Geometry check sheet. Reference: drawing and pictorial views, mm from the part's lowest x, y, z. A direction names the side the tool comes from. Coordinates: 2 decimals unless noted, no trailing zeros. Write each loop counter-clockwise with the first axis right and the second up, starting at its lowest first coordinate (ties: lowest second). Pieces come first, ordered by that corner, then holes. Notation, with made-up numbers: (45.5, 40) - (87.5, 40) arc R20 ccw to (87.5, 47) - close; hole circle Ø1 at (30.25, 74.25). An arc over 180 degrees is marked (long way). Answer as a JSON object with one key per item and string values. Group by question number.
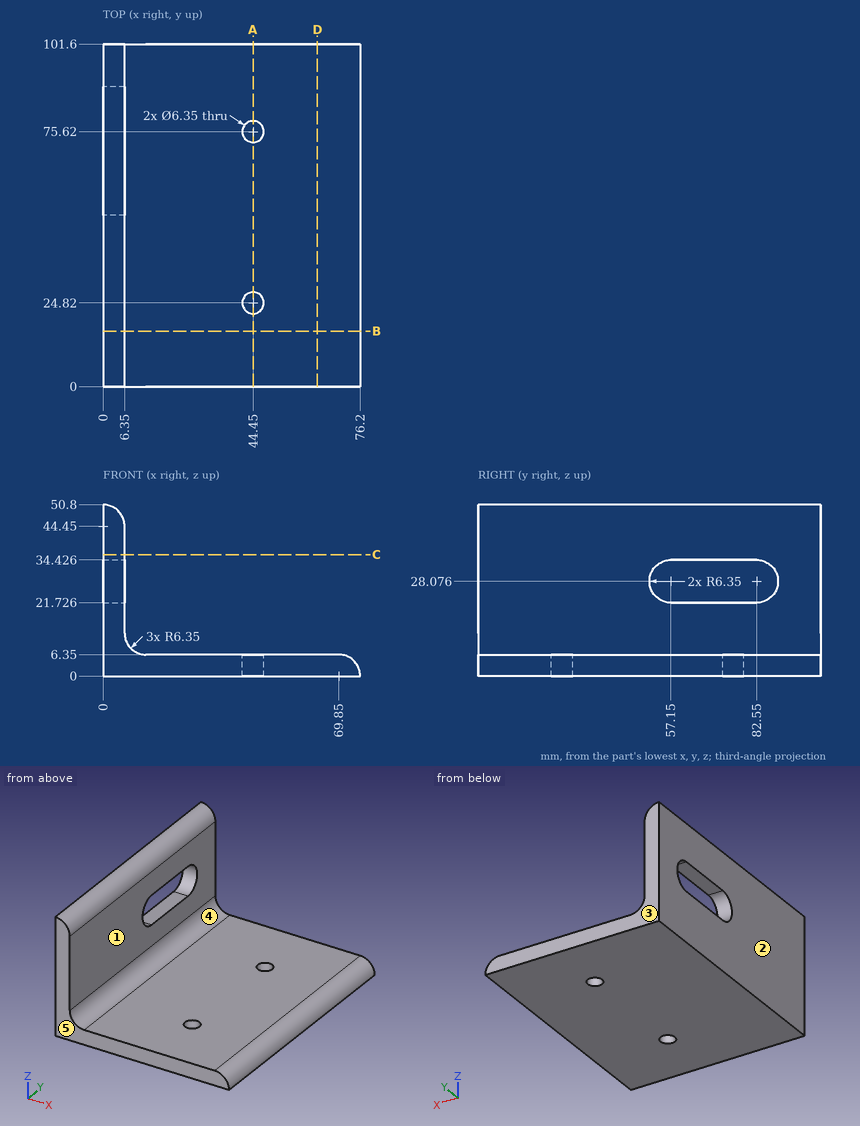
(1) Material ranges on L1, parallel to Y at x = 44.45, z = 4 (1 decimal); L2, parallel to X at y = 10.5, z = 17.5; L3, parallel to Z at x = 5.5, y = 43 (1 decimal), recorded low to high. Write a range as [from, to].
(2) Section check B-B (y = 16.5). Record the cut outline in (x, z).
(3) Section check C-C (z = 36). Record the cut outline in (x, y), and give its area (3 significant figures).
(4) Draft check along Y on the marked faces 3, 4 and 5. Enter one of: +Y half, -Y half, draft (parallel to the pull), parting line (faces both ways), or undercut.
(5) Section check D-D (x = 63.5). Record the cut outline in (y, z).
(6) Section check A-A (x = 44.45). Count the separate pieces of the cut face and the enclosed holes in it.
(7) Set-up check for the marked faces 1 and 2: record each of +Z, -Z, +X, -X, +Y, -Y from which the full face is reachable in a straight line by a thin tool's end or side.
(8) Gauge pin test, flat ends, axial feed: pin 1 (2 mm diameter, centred on x = 22.5, y = 34, fed in from +Z); pin 2 (4 mm diameter, centred on y = 89.5, z = 11, fed in from +X); pin 3 (5 mm diameter, centred on x = 3, y = 75.5, fed in from +Z). Record the tip position at first contact, or that the pin passes through.
Conclusion:
{
 "1": {"L1": "y = [0, 21.6], [28, 72.4], [78.8, 101.6]", "L2": "x = [0, 6.35]", "L3": "z = [0, 47.6]"},
 "2": {"outline": "(0, 0) - (76.2, 0) arc R6.35 ccw to (69.85, 6.35) - (12.7, 6.35) arc R6.35 cw to (6.35, 12.7) - (6.35, 44.45) arc R6.35 ccw to (0, 50.8) - close"},
 "3": {"outline": "(0, 0) - (6.35, 0) - (6.35, 101.6) - (0, 101.6) - close", "area": "645 mm^2"},
 "4": {"face 3": "+Y half", "face 4": "draft", "face 5": "-Y half"},
 "5": {"outline": "(0, 0) - (101.6, 0) - (101.6, 6.35) - (0, 6.35) - close"},
 "6": {"separate pieces": "3", "enclosed holes": "0"},
 "7": {"face 1": "+Z, +X, +Y, -Y", "face 2": "+Z, -Z, -X, +Y, -Y"},
 "8": {"pin 1": "stops at z = 6.35", "pin 2": "stops at x = 7.54", "pin 3": "stops at z = 50.78"}
}
